Autodesk Inventor part; units mm, degrees
ref_plane "Work Plane1" through (0, 12.7, 0) normal (0, 1, 0) x (-1, 0, 0)
ref_plane "YZ Plane" through (0, 0, 0) normal (1, 0, 0) x (0, 1, 0)
ref_plane "XY Plane" through (0, 0, 0) normal (0, 0, 1) x (1, 0, 0)
sketch "Sketch1" plane through (0, 0, 0) normal (0, 0, 1) x (1, 0, 0)
  circle A0 centre (0, 0) radius 12.7
  circle A1 centre (0, 0) radius 11.1125
  dimension "d0" = 25.4
  dimension "d1" = 22.225
extrude "Extrusion1" add sketch "Sketch1" along normal blind 393.7
ref_plane "Work Plane1" through (0, 12.7, 0) normal (0, 1, 0) x (-1, 0, 0)
sketch "Sketch2" plane through (0, 12.7, 0) normal (0, 1, 0) x (-1, 0, 0)
  line L0 (-12.7, 0) -> (-12.7, 393.7)
  line L1 (-12.7, 0) -> (12.7, 0)
  line L2 (12.7, 0) -> (12.7, 393.7)
  circle A0 centre (0, 12.7) radius 4.7625
  line L3 (0, 0) -> (0, 58.059) construction
  circle A1 centre (0, 95.25) radius 2.413
  dimension "d4" = 9.525
  dimension "d6" = 12.7
  dimension "d10" = 4.826
  dimension "d11" = 95.25
extrude "Extrusion2" cut sketch "Sketch2" against normal blind 25.4
properties part number "Polycarbonate Clamp Tube 1 in OD (8585K14)" material "Polycarbonate, Clear"
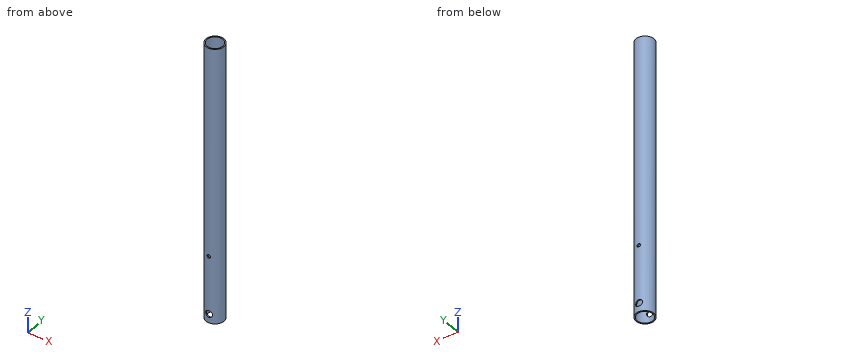
The listing builds one solid part. Answer for the finished solid, in the listing's coordinates (mm). Give positions to 0.01 mm unless a question says otherwise; leave off trailing zeros. Write each loop counter-clockwise with the first axis right and the second up, starting at its lowest first coordinate (ties: lowest second). Pieces come first, ordered by that corner, then holes.
1) Section A-A (y = 0) is taken. Write down the section's boundary in (x, z).
2) Given P1, Ø3, axis at x = 6, z = 59.5, coming from the -Y side; P2, Ø3, axis at y = -8, z = 102, coming from the -X side; P3, Ø3, axis at x = 9, z = 84.5, coming from the -Y side, each flat-ended and moving along its own axis, determine where each tip first touches the part or whether it passes through.
3) Section B-B (z = 12.7) is taken. Write down the section's boundary in (x, y) (1 decimal), and give its area (3 significant figures).
4) Find the intervals of material crossed by L1, parallel to Z at x = 0, y = -11.9; L2, parallel to Y at x = 1, z = 298; L3, parallel to X at y = -0.5, z = 23, in increasing order.
5) Section C-C (z = 280.5) is taken. Write down the section's boundary in (x, y) (1 decimal).
Response:
1. outline: (-12.7, 0) - (-11.11, 0) - (-11.11, 393.7) - (-12.7, 393.7) - close; (11.11, 0) - (12.7, 0) - (12.7, 393.7) - (11.11, 393.7) - close
2. P1: stops at y = -11.88
2. P2: stops at x = -10.91
2. P3: stops at y = -10.25
3. outline: (-4.8, -11.8) - (-4.8, -10) arc R11.1 cw to (-4.8, 10) - (-4.8, 11.8) arc R12.7 ccw to start; (4.8, -11.8) arc R12.7 ccw to (4.8, 11.8) - (4.8, 10) arc R11.1 cw to (4.8, -10) - close
3. area: 87.6 mm2
4. L1: z = 0 to 7.94, 17.46 to 92.84, 97.66 to 393.7
4. L2: y = -12.66 to -11.07, 11.07 to 12.66
4. L3: x = -12.69 to -11.1, 11.1 to 12.69
5. outline: circle Ø25.4 at (0, 0); hole circle Ø22.2 at (0, 0)
